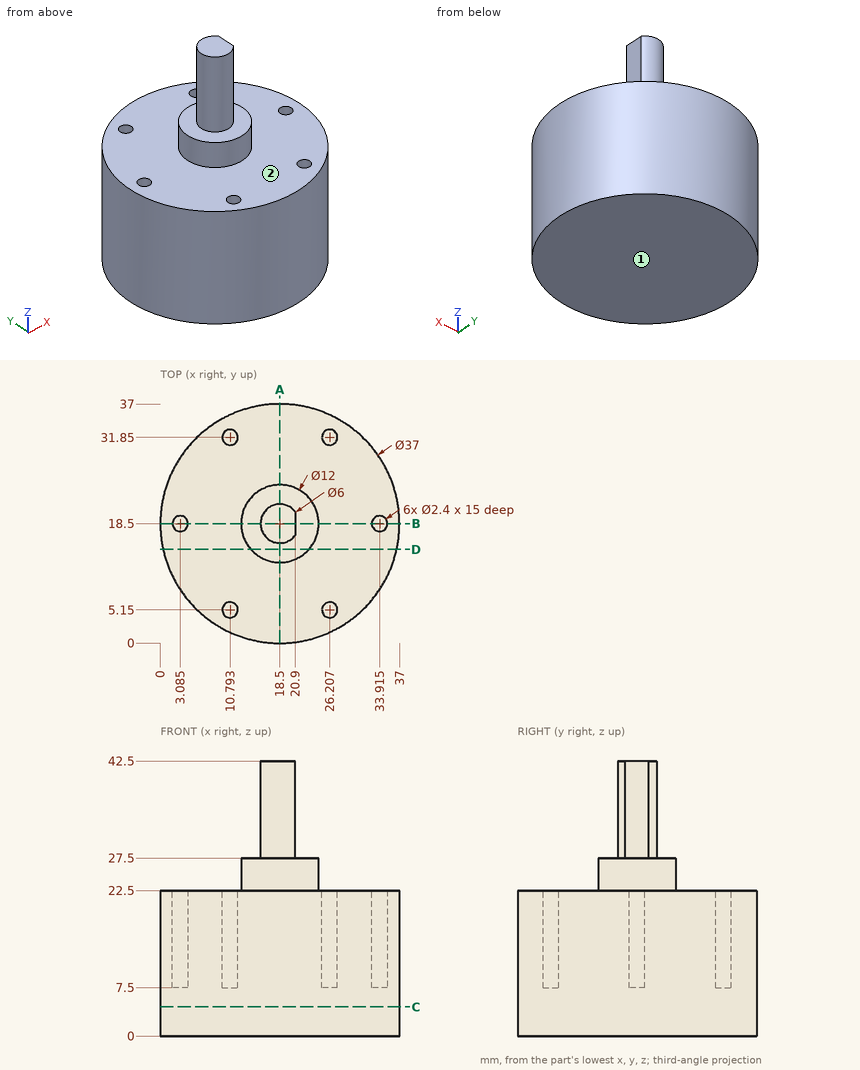
Check sheet for the drawn part. Datum: minimum x, y, z corner. Units: mm. A direction names the side the tool comes from. Coordinates: 2 decimals unless noted, no trailing zeros. Loops run counter-clockwise (first coordinate to the right, second up) from the corner with the lowest first, then second, coordinate; pieces in that order, holes last. Notation, with made-up numbers: (68, 60.5) -> (111, 60.5) arc R21 cw to (111, 96.5) -> close; hole circle Ø2 at (1.25, 68.5). An arc over 180 degrees is marked (long way). Write each question's results on one line, items separated by ' | '.
Item 1: Section check D-D, the plane y = 14.5. Enter the section's corners in (x, z).
Found:
outline: (0.44, 0) -> (36.56, 0) -> (36.56, 22.5) -> (22.97, 22.5) -> (22.97, 27.5) -> (14.03, 27.5) -> (14.03, 22.5) -> (0.44, 22.5) -> close
Item 2: Section check B-B, the plane y = 18.5. Enter the section's corners in (x, z) (1 decimal).
Found:
outline: (0, 0) -> (37, 0) -> (37, 22.5) -> (35.1, 22.5) -> (35.1, 7.5) -> (32.7, 7.5) -> (32.7, 22.5) -> (24.5, 22.5) -> (24.5, 27.5) -> (20.9, 27.5) -> (20.9, 42.5) -> (15.5, 42.5) -> (15.5, 27.5) -> (12.5, 27.5) -> (12.5, 22.5) -> (4.3, 22.5) -> (4.3, 7.5) -> (1.9, 7.5) -> (1.9, 22.5) -> (0, 22.5) -> close
Item 3: Section check A-A, the plane x = 18.5. Enter the section's corners in (y, z).
Found:
outline: (0, 0) -> (37, 0) -> (37, 22.5) -> (24.5, 22.5) -> (24.5, 27.5) -> (21.5, 27.5) -> (21.5, 42.5) -> (15.5, 42.5) -> (15.5, 27.5) -> (12.5, 27.5) -> (12.5, 22.5) -> (0, 22.5) -> close
Item 4: Material ranges on L1, parallel to Z at x = 5.5, y = 31; L2, parallel to Z at x = 16.5, y = 24; L3, parallel to Y at x = 18, z = 4, recorded low to high.
Found:
L1: z = 0 to 22.5 | L2: z = 0 to 27.5 | L3: y = 0.01 to 36.99
Item 5: Gauge pin test, flat ends, axial feed: pin 1 (1.5 mm diameter, centred on x = 33, z = 11, fed in from -Y) (1 decimal); pin 2 (1 mm diameter, centred on x = 32.5, z = 9.5, fed in from -Y); pin 3 (6 mm diameter, centred on x = 24.5, z = 24, fed in from -Y) (1 decimal); pin 4 (5 mm diameter, centred on x = 24, z = 35.5, fed in from +Y). Record the tip position at first contact, or that the pin passes through.
Found:
pin 1: stops at y = 6.1 | pin 2: stops at y = 5.85 | pin 3: stops at y = 0.3 | pin 4: passes through
Item 6: Section check C-C, the plane z = 4.5. Enter the section's corners in (x, y), plus the area to 3 significant figures.
Found:
outline: circle Ø37 at (18.5, 18.5) | area: 1,080 mm2
Item 7: Tool access check on the marked faces 1 and 2. Record the directions out of +Z, -Z, +X, -X, +Y, -Y that give a thin tool (end or side, any length) a straight path to the whole face; none if there is none.
Found:
face 1: -Z, +X, -X, +Y, -Y | face 2: +Z
